```python
from build123d import *

# Parameters (mm, degrees)
SKETCH1_W           = 12.7
SKETCH1_H           = 12.7
BOSS_EXTRUDE1_DEPTH = 12.7
SKETCH2_W           = 12.7
SKETCH2_H           = 12.7
SKETCH2_W_2         = 5.334
SKETCH2_H_2         = 2.794
BOSS_EXTRUDE2_DEPTH = 5.08
SKETCH3_W           = 6.858
SKETCH3_H           = 10.16
CUT_EXTRUDE1_DEPTH  = 9.525
SKETCH4_R           = 2.38125
CUT_EXTRUDE2_DEPTH  = 32.108519733
BOSS_EXTRUDE3_DEPTH = 12.7
SKETCH8_R           = 5.08
CUT_EXTRUDE5_DEPTH  = 91.094949376
FILLET2_R           = 6.35
SKETCH9_R           = 6.985
SKETCH9_W           = 80.922597298
SKETCH9_H           = 13.97
CUT_EXTRUDE6_DEPTH  = 2.032


with BuildPart() as part:
    # Sketch1 → Boss-Extrude1 (new body)
    with BuildSketch(Plane.XY):
        with Locations((-6.35, 6.35)):
            Rectangle(SKETCH1_W, SKETCH1_H)
    extrude(amount=BOSS_EXTRUDE1_DEPTH)

    # Sketch2 → Boss-Extrude2 (add)
    # profile 1 of 2: a face of its own
    with BuildSketch(Plane.ZY.offset(12.7)):
        with Locations((6.35, 19.05)):
            Rectangle(SKETCH2_W, SKETCH2_H)
        with Locations((6.35, 20.32)):
            Rectangle(SKETCH2_W_2, SKETCH2_H_2, mode=Mode.SUBTRACT)
    # profile 2 of 2: a face of its own
    with BuildSketch(Plane.ZY.offset(12.7)):
        with Locations((6.35, -6.35)):
            Rectangle(SKETCH2_W, SKETCH2_H)
        with Locations((6.35, -7.62)):
            Rectangle(SKETCH2_W_2, SKETCH2_H_2, mode=Mode.SUBTRACT)
    extrude(amount=-BOSS_EXTRUDE2_DEPTH)

    # Sketch3 → Cut-Extrude1 (cut)
    with BuildSketch(Plane.ZY.offset(12.7)):
        with Locations((6.35, 6.35)):
            Rectangle(SKETCH3_W, SKETCH3_H)
    extrude(amount=-CUT_EXTRUDE1_DEPTH, mode=Mode.SUBTRACT)

    # Sketch4 → Cut-Extrude2 (cut, through all)
    with BuildSketch(Plane.XY.offset(12.7)):
        with Locations((-7.9375, 6.35)):
            Circle(SKETCH4_R)
    extrude(amount=-CUT_EXTRUDE2_DEPTH, mode=Mode.SUBTRACT)

    # Sketch7 → Boss-Extrude3 (add)
    with BuildSketch(Plane(origin=(0, 12.7, 0), x_dir=(1, 0, 0), z_dir=(0, 1, 0))):
        Polygon((72.465692557, -41.838087105), (69.290692557, -47.337348419), (0, -7.332348419), (3.175, -1.833087105), align=None)
        Polygon((0, 0), (0, -7.332348419), (3.175, -1.833087105), align=None)
    extrude(amount=-BOSS_EXTRUDE3_DEPTH)

    # Sketch8 → Cut-Extrude5 (cut, through all)
    with BuildSketch(Plane(origin=(-3.175, 0, 5.499261314), x_dir=(0.8660254037844417, 0, 0.49999999999999495), z_dir=(-0.49999999999999495, 0, 0.8660254037844417))):
        with Locations((13.826174209, 6.35)):
            Circle(SKETCH8_R)
        with Locations((26.526174209, 6.35)):
            Circle(SKETCH8_R)
        with Locations((39.226174209, 6.35)):
            Circle(SKETCH8_R)
        with Locations((51.926174209, 6.35)):
            Circle(SKETCH8_R)
        with Locations((64.626174209, 6.35)):
            Circle(SKETCH8_R)
        with Locations((77.326174209, 6.35)):
            Circle(SKETCH8_R)
    extrude(amount=-CUT_EXTRUDE5_DEPTH, mode=Mode.SUBTRACT)

    # Fillet2
    fillet2_edges = [part.edges().sort_by_distance(p)[0] for p in [
        (70.878192557, 0, 44.587717762),
        (70.878192557, 12.7, 44.587717762),
    ]]
    fillet(fillet2_edges, radius=FILLET2_R - 0.0001)  # a hair under: the kernel refuses the full size

    # Sketch9 → Cut-Extrude6 (cut)
    with BuildSketch(Plane(origin=(0, 0, 0), x_dir=(-0.8660254037844417, 0, -0.4999999999999947), z_dir=(0.4999999999999947, 0, -0.8660254037844417))):
        with Locations((-13.826174209, 6.35)):
            Circle(SKETCH9_R)
        with Locations((-54.287472858, 6.35)):
            Rectangle(SKETCH9_W, SKETCH9_H)
    extrude(amount=-CUT_EXTRUDE6_DEPTH, mode=Mode.SUBTRACT)


solid = part.part
```
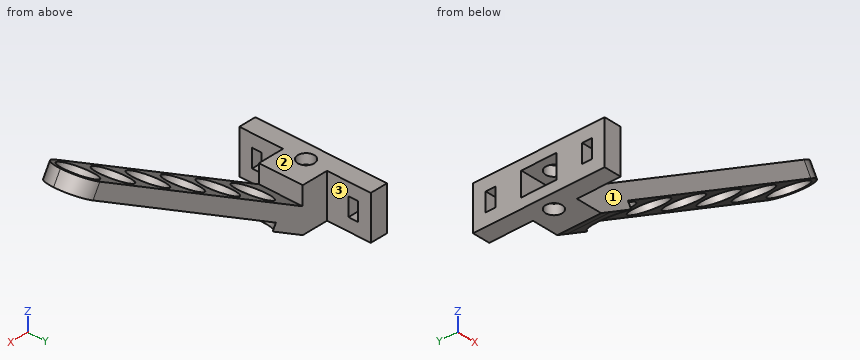
The listing builds one solid part. Answer for the finished solid, in the listing's coordinates (mm). Face numbers are marked on the shaded views. A direction names the side the tool comes from. Give positions to 0.01 mm unless a question says otherwise; leave off trailing zeros. Order: outer loops, then holes, each group sorted by start corner. A loop starts at its lowest first (then second) coordinate and runs counter-clockwise, first axis right, second up.
Item 1: Find the intervals of material crossed by probe 1 along X at (y, z) = (-11, 10.5); probe 2 along Y at (x, z) = (-0.5, 5.5); probe 3 along X at (y, z) = (6, 11), in increasing order.
From the geometry:
probe 1: x = -12.7 to -7.62
probe 2: y = 0 to 12.7
probe 3: x = -12.7 to -10.29, -5.58 to 0
Item 2: Which of the six approach directions +Z, -Z, +X, -X, +Y, -Y give full straight-line access (tool end or side, diameter ignored) to the marked faces 1, 2 and 3?
From the geometry:
face 1: +Z, -Z, +X, -Y
face 2: +Z, -X, +Y, -Y
face 3: +Z, -Z, +X, +Y
Item 3: The part is cut by section A-A, the plane y = 18. Give the vertices of the cut face in (x, z), and give its area (3 significant figures).
From the geometry:
outline: (-12.7, 0) - (-7.62, 0) - (-7.62, 12.7) - (-12.7, 12.7) - close
area: 64.5 mm2
Item 4: Given pin 1 Ø10.5 at (x, y) = (-6, 6) entering from +Z; pin 2 Ø3 at (x, y) = (-7.94, 6.35) entering from -Z; pin 3 Ø2 at (x, z) = (-7.5, 6.5) entering from +Y; pin 4 Ø6 at (y, z) = (3, 29) entering from -X, each flat-ended and moving along its own axis, determine where each tip first touches the part or whether it passes through.
From the geometry:
pin 1: stops at z = 12.7
pin 2: passes through
pin 3: stops at y = 25.4
pin 4: stops at x = 32.76
